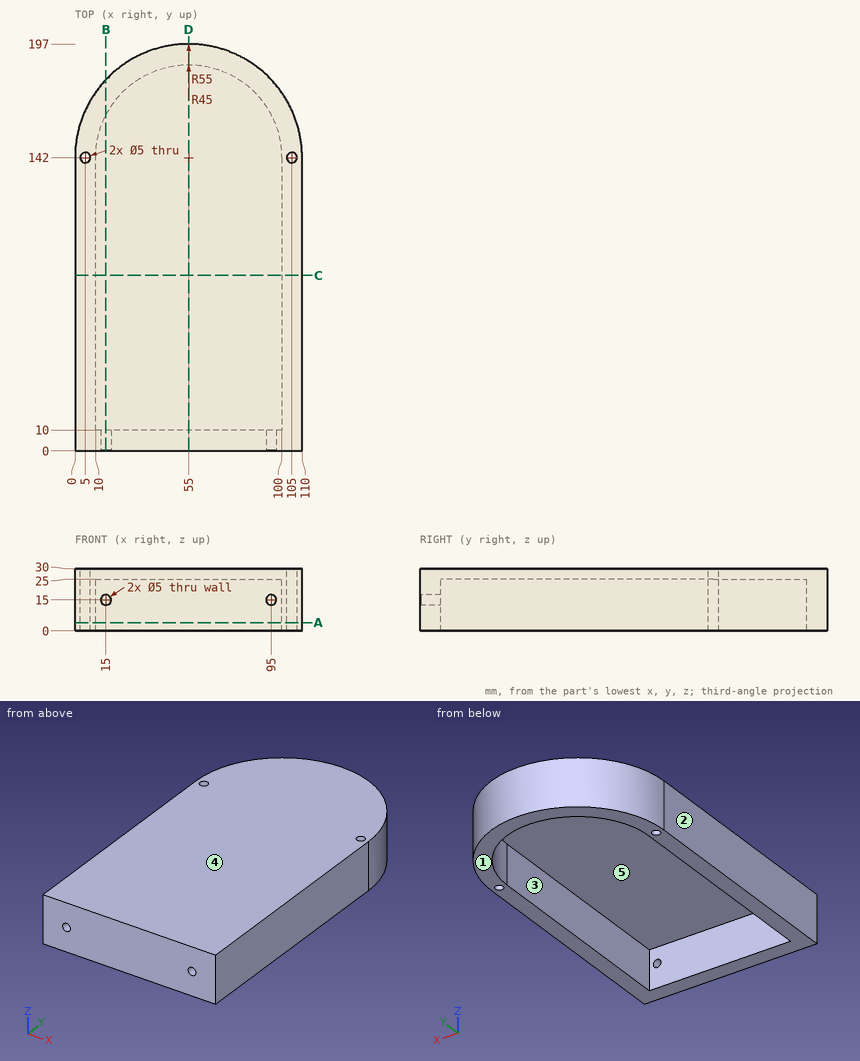
Check sheet for the drawn part. Datum: minimum x, y, z corner. Units: mm. A direction names the side the tool comes from. Coordinates: 2 decimals unless noted, no trailing zeros. Loops run counter-clockwise (first coordinate to the right, second up) from the corner with the lowest first, then second, coordinate; pieces in that order, holes last. Notation, with made-up numbers: (-23, 49.5) -> (3, 49.5) arc R19 cw to (3, 70.5) -> close; hole circle Ø1 at (69, 41). An arc over 180 degrees is marked (long way). Answer as CSV lines item,"result".
1) Cross-section at C-C, the plane y = 85. Record the cut outline in (x, z).
Found:
outline,"(0, 0) -> (10, 0) -> (10, 25) -> (100, 25) -> (100, 0) -> (110, 0) -> (110, 30) -> (0, 30) -> close"
2) Thickness scan on L1, parallel to X at y = 142, z = 19; L2, parallel to X at y = 127.5, z = 6; L3, parallel to X at y = 4, z = 15. Record the ranges inside material, lowest first. Write a range as from..to.
Found:
L1,"x = 0..2.5, 7.5..10, 100..102.5, 107.5..110"
L2,"x = 0..10, 100..110"
L3,"x = 0..12.5, 17.5..92.5, 97.5..110"
3) Release check for a two-part mould opening along X. For the marked faces 1, 2 and 3 record: +X half, -X half, draft (parallel to the pull), parting line (faces both ways), or undercut.
Found:
face 1,"draft"
face 2,"-X half"
face 3,"undercut"
4) Depth check by flat-ended pin: pin 1 (1.5 mm diameter, centred on x = 35.5, y = 43, fed in from -Z). Enter the tip coordinate at first touch or a pass-through.
Found:
pin 1,"stops at z = 25"
5) Cross-section at A-A, the plane z = 4. Record the cut outline in (x, y), then the cut area to 3 significant figures.
Found:
outline,"(0, 0) -> (110, 0) -> (110, 142) arc R55 ccw to (0, 142) -> close; hole circle Ø5 at (5, 142); hole (10, 10) -> (100, 10) -> (100, 142) arc R45 ccw to (10, 142) -> close; hole circle Ø5 at (105, 142)"
area,"5,270 mm2"
6) Cross-section at B-B, the plane x = 15. Record the cut outline in (y, z).
Found:
outline,"(0, 0) -> (10, 0) -> (10, 12.5) -> (0, 12.5) -> close; (0, 17.5) -> (10, 17.5) -> (10, 25) -> (162.62, 25) -> (162.62, 0) -> (179.75, 0) -> (179.75, 30) -> (0, 30) -> close"
7) Tool access check on the marked faces 4 and 5. Record the directions out of +Z, -Z, +X, -X, +Y, -Y that give a thin tool (end or side, any length) a straight path to the whole face; none if there is none.
Found:
face 4,"+Z, +X, -X, +Y, -Y"
face 5,"-Z"
8) Cross-section at D-D, the plane x = 55. Record the cut outline in (y, z).
Found:
outline,"(0, 0) -> (10, 0) -> (10, 25) -> (187, 25) -> (187, 0) -> (197, 0) -> (197, 30) -> (0, 30) -> close"
